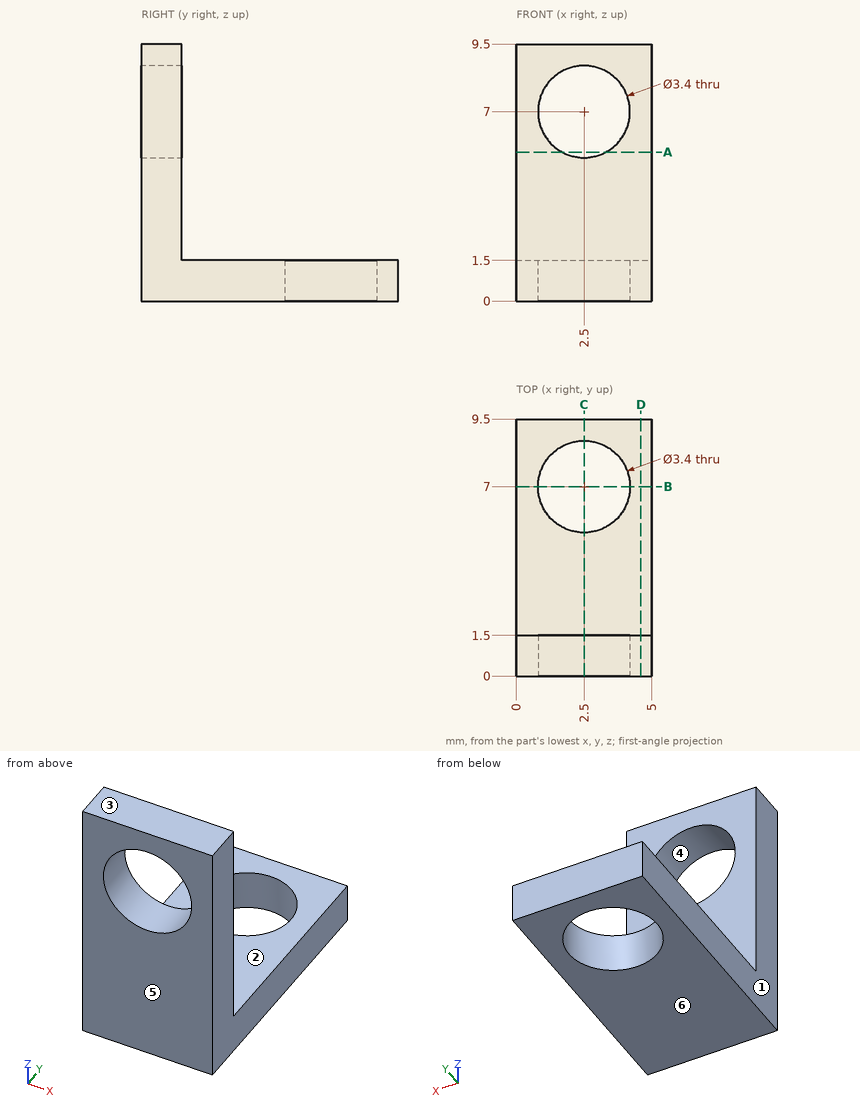
Study the drawing (mm; zero at the part's minimum x, y, z) and answer. A direction names the side the tool comes from. Coordinates: 2 decimals unless noted, no trailing zeros. Write each loop counter-clockwise with the first axis right and the second up, starting at its lowest first coordinate (ties: lowest second). Pieces come first, ordered by that corner, then holes. Notation, with made-up numbers: (51, 82.25) -> (102, 82.25) arc R27 cw to (102, 103.25) -> close; hole circle Ø9 at (-10, 83). An arc over 180 degrees is marked (long way). Write each question's results on one line, items separated by ' | '. Start each with the question number.
1) A tool of negligible diameter and unlimited length cuts with its end or side. For the marked faces 1 and 2, from which of +Z, -Z, +X, -X, +Y, -Y can it reach the whole face along a straight path? Write none if from no direction.
2) Straight lines are drawn through the part: probe 1 along Y at (x, z) = (2.5, 0.6); probe 2 along Z at (x, y) = (0.5, 3). For each, find the intervals that lie inside material, in ascending order.
3) A cutting plane is placed at D-D (x = 4.6). Determine the outline of the cut face in (y, z).
4) A cutting plane is placed at C-C (x = 2.5). Determine the outline of the cut face in (y, z), then the cut area to 4 significant figures.
5) A cutting plane is placed at B-B (y = 7). Determine the outline of the cut face in (x, z), then the cut area to 3 significant figures.
6) For a pull along Z with two mould halves and no side action, classify the marked faces 3, 4, 5 and 6 as +Z half, -Z half, draft (parallel to the pull), parting line (faces both ways), or undercut.
7) Flat-ended cylindrical pins translate along their axes: pin 1 Ø1 at (x, z) = (4.5, 7) entering from +Y; pin 2 Ø1.5 at (x, y) = (1, 6) entering from +Z; pin 3 Ø3 at (x, z) = (2.5, 7) entering from -Y. Find the tip coordinate at first contact, or state that the pin passes through.
8) A cutting plane is placed at A-A (z = 5.5). Determine the outline of the cut face in (x, y), then the cut area to 3 significant figures.
Values follow:
1) face 1: +Z, -Z, -X, +Y, -Y | face 2: +Z, +X, -X, +Y
2) probe 1: 0 to 5.3, 8.7 to 9.5 | probe 2: 0 to 1.5
3) outline: (0, 0) -> (9.5, 0) -> (9.5, 1.5) -> (1.5, 1.5) -> (1.5, 9.5) -> (0, 9.5) -> close
4) outline: (0, 0) -> (5.3, 0) -> (5.3, 1.5) -> (1.5, 1.5) -> (1.5, 5.3) -> (0, 5.3) -> close; (0, 8.7) -> (1.5, 8.7) -> (1.5, 9.5) -> (0, 9.5) -> close; (8.7, 0) -> (9.5, 0) -> (9.5, 1.5) -> (8.7, 1.5) -> close | area: 16.05 mm²
5) outline: (0, 0) -> (0.8, 0) -> (0.8, 1.5) -> (0, 1.5) -> close; (4.2, 0) -> (5, 0) -> (5, 1.5) -> (4.2, 1.5) -> close | area: 2.40 mm²
6) face 3: +Z half | face 4: undercut | face 5: draft | face 6: -Z half
7) pin 1: y = 1.5 | pin 2: z = 1.5 | pin 3: through
8) outline: (0, 0) -> (1.7, 0) -> (1.7, 1.5) -> (0, 1.5) -> close; (3.3, 0) -> (5, 0) -> (5, 1.5) -> (3.3, 1.5) -> close | area: 5.10 mm²
